Could you check a few things on this model? Use its own coordinates, in mm. A direction names the side the tool comes from. Coordinates: 2 decimals unless noted, no trailing zeros. Loops run counter-clockwise (first coordinate to the right, second up) from the corner with the lowest first, then second, coordinate; pieces in that order, holes last. Notation, with made-up numbers: M 77.5,-6 L 114.5,-6 A18 cw 114.5,21 Z; hole C 42,32 d11. An arc over 180 degrees is marked long. Write each question's results on one line, items separated by ' | '.
```python
from build123d import *

# Parameters (mm, degrees)
SKETCH1_W               = 165.1
SKETCH1_H               = 92.075
BOSS_EXTRUDE1_DEPTH     = 2.54
SKETCH2_R               = 1.905
SKETCH2_R_2             = 1.2192
CUT_EXTRUDE1_DEPTH      = 2.54
SKETCH4_W               = 2.54
SKETCH4_H               = 92.075
BOSS_EXTRUDE3_DEPTH     = 203.2
SKETCH6_W               = 38.1
SKETCH6_H               = 2.54
BOSS_EXTRUDE4_DEPTH     = 160.02
SKETCH7_W               = 160.02
SKETCH7_H               = 50.8
BOSS_EXTRUDE5_DEPTH     = 2.54
CUT_EXTRUDE2_DEPTH      = 1
CUT_EXTRUDE2_DEPTH_BACK = 166.1


with BuildPart() as part:
    # Sketch1 → Boss-Extrude1 (new body)
    with BuildSketch(Plane.XY):
        with Locations((259.660273445, 73.209654415)):
            Rectangle(SKETCH1_W, SKETCH1_H)
    extrude(amount=-BOSS_EXTRUDE1_DEPTH)

    # Sketch2 → Cut-Extrude1 (cut)
    with BuildSketch(Plane.XY):
        with Locations((188.032273445, 41.815254415)):
            Circle(SKETCH2_R)
        with Locations((226.132273445, 104.604054415)):
            Circle(SKETCH2_R)
        with Locations((188.032273445, 104.604054415)):
            Circle(SKETCH2_R)
        with Locations((188.032273445, 36.278054415)):
            Circle(SKETCH2_R_2)
        with Locations((188.032273445, 30.715454415)):
            Circle(SKETCH2_R_2)
        with Locations((226.132273445, 41.815254415)):
            Circle(SKETCH2_R)
        with Locations((226.132273445, 36.278054415)):
            Circle(SKETCH2_R_2)
        with Locations((226.132273445, 30.715454415)):
            Circle(SKETCH2_R_2)
        with Locations((226.132273445, 110.141254415)):
            Circle(SKETCH2_R_2)
        with Locations((226.132273445, 115.703854415)):
            Circle(SKETCH2_R_2)
        with Locations((188.032273445, 110.141254415)):
            Circle(SKETCH2_R_2)
        with Locations((188.032273445, 115.703854415)):
            Circle(SKETCH2_R_2)
        with Locations((240.610273445, 41.815254415)):
            Circle(SKETCH2_R)
        with Locations((278.710273445, 104.604054415)):
            Circle(SKETCH2_R)
        with Locations((240.610273445, 104.604054415)):
            Circle(SKETCH2_R)
        with Locations((240.610273445, 36.278054415)):
            Circle(SKETCH2_R_2)
        with Locations((240.610273445, 30.715454415)):
            Circle(SKETCH2_R_2)
        with Locations((278.710273445, 41.815254415)):
            Circle(SKETCH2_R)
        with Locations((278.710273445, 36.278054415)):
            Circle(SKETCH2_R_2)
        with Locations((278.710273445, 30.715454415)):
            Circle(SKETCH2_R_2)
        with Locations((278.710273445, 110.141254415)):
            Circle(SKETCH2_R_2)
        with Locations((278.710273445, 115.703854415)):
            Circle(SKETCH2_R_2)
        with Locations((240.610273445, 110.141254415)):
            Circle(SKETCH2_R_2)
        with Locations((240.610273445, 115.703854415)):
            Circle(SKETCH2_R_2)
        with Locations((293.188273445, 41.815254415)):
            Circle(SKETCH2_R)
        with Locations((331.288273445, 104.604054415)):
            Circle(SKETCH2_R)
        with Locations((293.188273445, 104.604054415)):
            Circle(SKETCH2_R)
        with Locations((293.188273445, 36.278054415)):
            Circle(SKETCH2_R_2)
        with Locations((293.188273445, 30.715454415)):
            Circle(SKETCH2_R_2)
        with Locations((331.288273445, 41.815254415)):
            Circle(SKETCH2_R)
        with Locations((331.288273445, 36.278054415)):
            Circle(SKETCH2_R_2)
        with Locations((331.288273445, 30.715454415)):
            Circle(SKETCH2_R_2)
        with Locations((331.288273445, 110.141254415)):
            Circle(SKETCH2_R_2)
        with Locations((331.288273445, 115.703854415)):
            Circle(SKETCH2_R_2)
        with Locations((293.188273445, 110.141254415)):
            Circle(SKETCH2_R_2)
        with Locations((293.188273445, 115.703854415)):
            Circle(SKETCH2_R_2)
        Polygon((191.334273445, 115.881654415), (222.830273445, 115.881654415), (222.830273445, 100.641654415), (227.656273445, 100.641654415), (227.656273445, 45.777654415), (222.830273445, 45.777654415), (222.830273445, 30.537654415), (191.334273445, 30.537654415), (191.334273445, 45.777654415), (186.508273445, 45.777654415), (186.508273445, 100.641654415), (191.334273445, 100.641654415), align=None)
        Polygon((243.912273445, 115.881654415), (275.408273445, 115.881654415), (275.408273445, 100.641654415), (280.234273445, 100.641654415), (280.234273445, 45.777654415), (275.408273445, 45.777654415), (275.408273445, 30.537654415), (243.912273445, 30.537654415), (243.912273445, 45.777654415), (239.086273445, 45.777654415), (239.086273445, 100.641654415), (243.912273445, 100.641654415), align=None)
        Polygon((296.490273445, 115.881654415), (327.986273445, 115.881654415), (327.986273445, 100.641654415), (332.812273445, 100.641654415), (332.812273445, 45.777654415), (327.986273445, 45.777654415), (327.986273445, 30.537654415), (296.490273445, 30.537654415), (296.490273445, 45.777654415), (291.664273445, 45.777654415), (291.664273445, 100.641654415), (296.490273445, 100.641654415), align=None)
    extrude(amount=-CUT_EXTRUDE1_DEPTH, mode=Mode.SUBTRACT)

    # Sketch4 → Boss-Extrude3 (add)
    with BuildSketch(Plane(origin=(0, 0, -2.54), x_dir=(-1, 0, 0), z_dir=(0, 0, -1))):
        with Locations((-340.940273445, 73.209654415)):
            Rectangle(SKETCH4_W, SKETCH4_H)
        with Locations((-178.380273445, 73.209654415)):
            Rectangle(SKETCH4_W, SKETCH4_H)
    extrude(amount=BOSS_EXTRUDE3_DEPTH)

    # Sketch6 → Boss-Extrude4 (add)
    with BuildSketch(Plane.ZY.offset(-339.670273445)):
        with Locations((-186.69, 28.442154415)):
            Rectangle(SKETCH6_W, SKETCH6_H)
    extrude(amount=BOSS_EXTRUDE4_DEPTH)

    # Sketch7 → Boss-Extrude5 (add)
    with BuildSketch(Plane.XZ.offset(-27.172154415)):
        with Locations((259.660273445, -100.037339466)):
            Rectangle(SKETCH7_W, SKETCH7_H)
    extrude(amount=-BOSS_EXTRUDE5_DEPTH)

    # Sketch8 → Cut-Extrude2 (cut, two sides)
    with BuildSketch(Plane(origin=(342.210273445, 0, 0), x_dir=(0, 0, -1), z_dir=(1, 0, 0))) as cut_extrude2_sk:
        Polygon((205.74, 119.247154415), (50.692993011, 119.247154415), (107.781148805, 52.572154415), (205.74, 52.572154415), align=None)
    extrude(amount=CUT_EXTRUDE2_DEPTH, mode=Mode.SUBTRACT)
    extrude(cut_extrude2_sk.sketch, amount=-CUT_EXTRUDE2_DEPTH_BACK, mode=Mode.SUBTRACT)


solid = part.part
```
(1) Imagine slicing it at D-D, the plane z = -170. List the corners of the cut face in (x, y) for me.
Reported:
outline: M 177.11,27.17 L 342.21,27.17 L 342.21,52.57 L 339.67,52.57 L 339.67,29.71 L 179.65,29.71 L 179.65,52.57 L 177.11,52.57 Z
(2) Please list where these lines run through material, in increasing order: probe 1 along X at (y, z) = (60.5, -23.5); probe 2 along Y at (x, z) = (298.5, -113); probe 3 along Z at (x, y) = (232, 41.5). Write a range as from..to.
Reported:
probe 1: x = 177.11..179.65, 339.67..342.21 | probe 2: y = 27.17..29.71 | probe 3: z = -2.54..0
(3) Imagine slicing it at A-A, the plane z = -44. List the corners of the cut face in (x, y) for me.
Reported:
outline: M 177.11,27.17 L 179.65,27.17 L 179.65,119.25 L 177.11,119.25 Z; M 339.67,27.17 L 342.21,27.17 L 342.21,119.25 L 339.67,119.25 Z
(4) Which directions (+Z, -Z, +X, -X, +Y, -Y) give clear straight access to the entire face, cutting with the end or side of a thin tool? Please do faces 4 (the flat face through (261, 29.712, -187)), 5 (the flat face through (178.398, 86.376, -78.837)).
Reported:
face 4: -Z, +Y | face 5: -Z, +X, -X, +Y
(5) Will these pins go through, and if not, where does the flat tip stop? P1, Ø12, axis at x = 212.5, z = -133, coming from the +Y side; P2, Ø3, axis at x = 226.13, y = 115.7, coming from the -Z side; P3, Ø6, axis at x = 238.5, y = 85.5, coming from the +Z side; P4, Ø2, axis at x = 341, z = -152, coming from the +Y side.
Reported:
P1: passes through | P2: stops at z = -2.54 | P3: stops at z = 0 | P4: stops at y = 52.57
(6) If we mould it in two halves opening along X, with no side actions, what happens to faces 1 (the flat face through (340.958, 86.376, -78.837)), 2 (the flat face through (259, 29.712, -100)), 3 (the flat face through (342.21, 62, -79))? For each: released by +X, released by -X, zero draft, split by the parting line, or undercut.
Reported:
face 1: zero draft | face 2: undercut | face 3: released by +X
(7) Imagine slicing it at B-B, the plane y = 64.5. List the corners of the cut face in (x, z) for me, and give its area (3 significant figures).
Reported:
outline: M 177.11,-97.57 L 179.65,-97.57 L 179.65,-2.54 L 186.51,-2.54 L 186.51,0 L 177.11,0 Z; M 227.66,-2.54 L 239.09,-2.54 L 239.09,0 L 227.66,0 Z; M 280.23,-2.54 L 291.66,-2.54 L 291.66,0 L 280.23,0 Z; M 332.81,-2.54 L 339.67,-2.54 L 339.67,-97.57 L 342.21,-97.57 L 342.21,0 L 332.81,0 Z | area: 589 mm2
(8) Imagine slicing it at C-C, the plane x = 271.5. List the corners of the cut face in (y, z) for me.
Reported:
outline: M 27.17,-205.74 L 29.71,-205.74 L 29.71,-167.64 L 27.17,-167.64 Z; M 27.17,-125.44 L 29.71,-125.44 L 29.71,-74.64 L 27.17,-74.64 Z; M 27.17,-2.54 L 30.54,-2.54 L 30.54,0 L 27.17,0 Z; M 115.88,-2.54 L 119.25,-2.54 L 119.25,0 L 115.88,0 Z
